Build history of the part. All positions in model axes, mm. A direction names the side the tool comes from. Coordinates: 2 decimals unless noted, no trailing zeros. Loops run counter-clockwise (first coordinate to the right, second up) from the corner with the lowest first, then second, coordinate; pieces in that order, holes last. Notation, with made-up numbers: (82.25, 6) - (112.25, 6) arc R25 cw to (112.25, 42) - close; hole circle Ø8 at (-31.75, -6.5). An arc over 180 degrees is marked (long way). One line per item, written item: value.
```python
from build123d import *

# Parameters (mm, degrees)
SKETCH_1_W          = 160
SKETCH_1_H          = 55
EXTRUDE_1_DEPTH     = 5
EXTRUDE_2_DEPTH     = 55
FILLET_1_R          = 27.5
CUT_EXTRUDE_1_REACH = 113.608
SKETCH_3_R          = 6.5
SKETCH_4_R          = 1.6
CUT_EXTRUDE_2_DEPTH = 10
CHAMFER_1_SIZE      = 8
CHAMFER_2_SIZE      = 8
EXTRUDE_5_DEPTH     = 5
CHAMFER_3_SIZE      = 1
SKETCH_7_R          = 2.1
CUT_EXTRUDE_3_DEPTH = 5


# Some blends are built 0.0001 mm under size
with BuildPart() as part:
    # 草图1 → 凸台-拉伸1 (new body)
    with BuildSketch(Plane(origin=(0, 0, 0), x_dir=(1, 0, 0), z_dir=(0, 1, 0))):
        Rectangle(SKETCH_1_W, SKETCH_1_H)
    extrude(amount=EXTRUDE_1_DEPTH)

    # 草图2 → 凸台-拉伸2 (add)
    with BuildSketch(Plane(origin=(0, 5, 0), x_dir=(1, 0, 0), z_dir=(0, 1, 0))):
        Polygon((10, 0), (10, 27.5), (15, 27.5), (15, -27.5), (10, -27.5), align=None)
    extrude(amount=EXTRUDE_2_DEPTH)

    # 圆角1
    fillet_1_edges = [part.edges().sort_by_distance(p)[0] for p in [
        (12.5, 60, -27.5),
        (12.5, 60, 27.5),
    ]]
    fillet(fillet_1_edges, radius=FILLET_1_R - 0.0001)  # a hair under: the kernel refuses the full size

    # 草图3 → 切除-拉伸1 (cut, up to next)
    with BuildSketch(Plane.ZY.offset(-10), mode=Mode.PRIVATE) as cut_extrude_1_sk1:
        with Locations((0, 40)):
            Circle(SKETCH_3_R)
    cut_extrude_1_tool1 = extrude(cut_extrude_1_sk1.sketch, amount=-CUT_EXTRUDE_1_REACH, mode=Mode.PRIVATE) & part.part
    add(cut_extrude_1_tool1.solids().sort_by_distance((10, 40, 0))[0], mode=Mode.SUBTRACT)

    # 草图4 → 切除-拉伸2 (cut)
    with BuildSketch(Plane.ZY.offset(-10)):
        with Locations((15.5, 33)):
            Circle(SKETCH_4_R)
        with Locations((7.75, 19.576606241)):
            Circle(SKETCH_4_R)
        with Locations((-7.75, 19.576606241)):
            Circle(SKETCH_4_R)
        with Locations((-15.5, 33)):
            Circle(SKETCH_4_R)
        with Locations((-7.75, 46.423393759)):
            Circle(SKETCH_4_R)
        with Locations((7.75, 46.423393759)):
            Circle(SKETCH_4_R)
    extrude(amount=-CUT_EXTRUDE_2_DEPTH, mode=Mode.SUBTRACT)

    # 倒角1
    chamfer_1_edges = [part.edges().sort_by_distance(p)[0] for p in [
        (10, 5, 0),
    ]]
    chamfer(chamfer_1_edges, length=CHAMFER_1_SIZE)

    # 倒角2
    chamfer_2_edges = [part.edges().sort_by_distance(p)[0] for p in [
        (15, 5, 0),
    ]]
    chamfer(chamfer_2_edges, length=CHAMFER_2_SIZE)

    # 草图6 → 凸台-拉伸5 (add)
    with BuildSketch(Plane.XY.offset(27.5)):
        Polygon((10, 5), (10, 32.5), (-17.5, 5), align=None)
        Polygon((15, 32.5), (15, 5), (42.5, 5), align=None)
    extrude_5 = extrude(amount=-EXTRUDE_5_DEPTH)

    # 镜向1: 凸台-拉伸5 across plane
    add(extrude_5.mirror(Plane.XY))

    # 倒角3
    # the kernel refuses this chamfer: 1 mm, written as the material it takes off along each edge
    with BuildSketch(Plane(origin=(10, 32.5001, 0.0001), x_dir=(0, -0.09341724291060717, 0.9956270480089322), z_dir=(0, -0.9956270480089322, -0.09341724291060717))) as chamfer_3_piece_1_section:
        Polygon((27.4999 - CHAMFER_3_SIZE, 0), (27.4999, -CHAMFER_3_SIZE), (27.4999, 0), align=None)
    chamfer_3_piece_1 = revolve(axis=Axis((10, 32.5001, 0.0001), (-1, 0, 0)), revolution_arc=100.720458749, mode=Mode.PRIVATE)
    chamfer_3_piece_1 = split(chamfer_3_piece_1, bisect_by=Plane(origin=(20.22926311, 42.72926311, 18.191765192), z_dir=(-0.7071067811865475, 0.7071067811865477, 0)), keep=Keep.TOP, mode=Mode.PRIVATE)
    add(chamfer_3_piece_1, mode=Mode.SUBTRACT)
    with BuildSketch(Plane(origin=(10, 32.5001, -0.0001), x_dir=(0, -0.09341724291060717, -0.9956270480089322), z_dir=(0, -0.9956270480089322, 0.09341724291060717))) as chamfer_3_piece_2_section:
        Polygon((27.4999, CHAMFER_3_SIZE), (27.4999 - CHAMFER_3_SIZE, 0), (27.4999, 0), align=None)
    chamfer_3_piece_2 = revolve(axis=Axis((10, 32.5001, -0.0001), (1, 0, 0)), revolution_arc=100.720458749, mode=Mode.PRIVATE)
    chamfer_3_piece_2 = split(chamfer_3_piece_2, bisect_by=Plane(origin=(20.397792602, 42.897792602, -19.088683077), z_dir=(-0.7071067811865475, 0.7071067811865477, 0)), keep=Keep.TOP, mode=Mode.PRIVATE)
    add(chamfer_3_piece_2, mode=Mode.SUBTRACT)
    with BuildSketch(Plane(origin=(15, 32.5001, 0.0001), x_dir=(0, -0.09341724291060717, 0.9956270480089322), z_dir=(0, -0.9956270480089322, -0.09341724291060717))) as chamfer_3_piece_3_section:
        Polygon((27.4999 - CHAMFER_3_SIZE, 0), (27.4999, CHAMFER_3_SIZE), (27.4999, 0), align=None)
    chamfer_3_piece_3 = revolve(axis=Axis((15, 32.5001, 0.0001), (-1, 0, 0)), revolution_arc=100.720458749, mode=Mode.PRIVATE)
    chamfer_3_piece_3 = split(chamfer_3_piece_3, bisect_by=Plane(origin=(4.77073689, 42.72926311, 18.191765192), z_dir=(0.7071067811865476, 0.7071067811865476, 0)), keep=Keep.TOP, mode=Mode.PRIVATE)
    add(chamfer_3_piece_3, mode=Mode.SUBTRACT)
    with BuildSketch(Plane(origin=(15, 32.5001, -0.0001), x_dir=(0, -0.09341724291060717, -0.9956270480089322), z_dir=(0, -0.9956270480089322, 0.09341724291060717))) as chamfer_3_piece_4_section:
        Polygon((27.4999 - CHAMFER_3_SIZE, 0), (27.4999, -CHAMFER_3_SIZE), (27.4999, 0), align=None)
    chamfer_3_piece_4 = revolve(axis=Axis((15, 32.5001, -0.0001), (1, 0, 0)), revolution_arc=100.720458749, mode=Mode.PRIVATE)
    chamfer_3_piece_4 = split(chamfer_3_piece_4, bisect_by=Plane(origin=(4.77073689, 42.72926311, -18.191765192), z_dir=(0.7071067811865476, 0.7071067811865476, 0)), keep=Keep.TOP, mode=Mode.PRIVATE)
    add(chamfer_3_piece_4, mode=Mode.SUBTRACT)

    # 草图7 → 切除-拉伸3 (cut)
    with BuildSketch(Plane(origin=(0, 0, 0), x_dir=(-1, 0, 0), z_dir=(0, -1, 0))):
        with Locations(Location((50, -15, 0), (0, 0, 90))):
            Circle(SKETCH_7_R)
        with Locations(Location((25, -15, 0), (0, 0, 90))):
            Circle(SKETCH_7_R)
        with Locations(Location((-30, -15, 0), (0, 0, 90))):
            Circle(SKETCH_7_R)
        with Locations(Location((-55, -15, 0), (0, 0, 90))):
            Circle(SKETCH_7_R)
        with Locations(Location((-55, 15, 0), (0, 0, 270))):
            Circle(SKETCH_7_R)
        with Locations(Location((-30, 15, 0), (0, 0, 270))):
            Circle(SKETCH_7_R)
        with Locations(Location((25, 15, 0), (0, 0, 270))):
            Circle(SKETCH_7_R)
        with Locations(Location((50, 15, 0), (0, 0, 270))):
            Circle(SKETCH_7_R)
    extrude(amount=-CUT_EXTRUDE_3_DEPTH, mode=Mode.SUBTRACT)


solid = part.part
```
Item 1: Tool access for faces 1 (the face through (12.53, 51.73, -19.66)), 2 (the face through (10, 31, 0)): list every direction of +Z, -Z, +X, -X, +Y, -Y with a clear straight run to the whole face (end or side of a thin tool).
Check result:
face 1: -Z, +X, -X, +Y
face 2: -X, +Y
Item 2: Cut at B-B, the plane y = 24. Write the cut outline in (x, z), then the cut area to 3 significant figures.
Check result:
outline: (1.5, -27.5) - (23.5, -27.5) - (23.5, -22.5) - (15, -22.5) - (15, 22.5) - (23.5, 22.5) - (23.5, 27.5) - (1.5, 27.5) - (1.5, 22.5) - (10, 22.5) - (10, -22.5) - (1.5, -22.5) - close
area: 445 mm^2
Item 3: Cut at A-A, the plane x = -50. Write the cut outline in (y, z).
Check result:
outline: (0, -27.5) - (5, -27.5) - (5, -17.1) - (0, -17.1) - close; (0, -12.9) - (5, -12.9) - (5, 12.9) - (0, 12.9) - close; (0, 17.1) - (5, 17.1) - (5, 27.5) - (0, 27.5) - close
Item 4: Probe probe 1 along X at (y, z) = (2.55, 15); probe 2 along Y at (x, z) = (-26.5, -6); probe 3 along X at (y, z) = (49, -15). List the from-to ranges inside material, lowest first. Write a range as from..to.
Check result:
probe 1: x = -80..-52.1, -47.9..-27.1, -22.9..27.9, 32.1..52.9, 57.1..80
probe 2: y = 0..5
probe 3: x = 10..15
Item 5: Cut at C-C, the plane x = 30. Write the cut outline in (y, z).
Check result:
outline: (0, -27.5) - (17.5, -27.5) - (17.5, -22.5) - (5, -22.5) - (5, -17.1) - (0, -17.1) - close; (0, -12.9) - (5, -12.9) - (5, 12.9) - (0, 12.9) - close; (0, 17.1) - (5, 17.1) - (5, 22.5) - (17.5, 22.5) - (17.5, 27.5) - (0, 27.5) - close
Item 6: Drop flat-ended pins along their axis: P1, Ø1.9, axis at y = 33, z = 15.5, coming from the +X side; P2, Ø12, axis at y = 42, z = -11.5, coming from the -X side; P3, Ø4, axis at y = 19.58, z = -7.75, coming from the +X side; P4, Ø6, axis at x = -38.5, z = -14.5, coming from the +Y side. Give the stop position or say it passes through.
Check result:
P1: passes through
P2: stops at x = 10
P3: stops at x = 15
P4: stops at y = 5
Item 7: Pull direction X, two halves, no side cores. Call faces 3 (the face through (27.95, 2.46, 15.46)), 4 (the face through (15, 31, 0)), 5 (the face through (-40, 5, 0)), 6 (the face through (52.95, 2.46, 15.46)): released by +X, released by -X, zero draft, split by the parting line, or undercut.
Check result:
face 3: undercut
face 4: released by +X
face 5: zero draft
face 6: undercut
